The listing builds one solid part. Answer for the finished solid, in the listing's coordinates (mm). Face numbers are marked on the shaded views. A direction names the side the tool comes from. Give positions to 0.01 mm unless a question says otherwise; leave off trailing zeros. Loops run counter-clockwise (first coordinate to the right, second up) from the corner with the lowest first, then second, coordinate; pieces in that order, holes last. Notation, with made-up numbers: (-9.75, -36) - (38.25, -36) arc R30 cw to (38.25, -3) - close; hole circle Ø4 at (14, 28.25). An arc over 180 degrees is marked (long way). One line per item, written item: value. Start each with the question number.
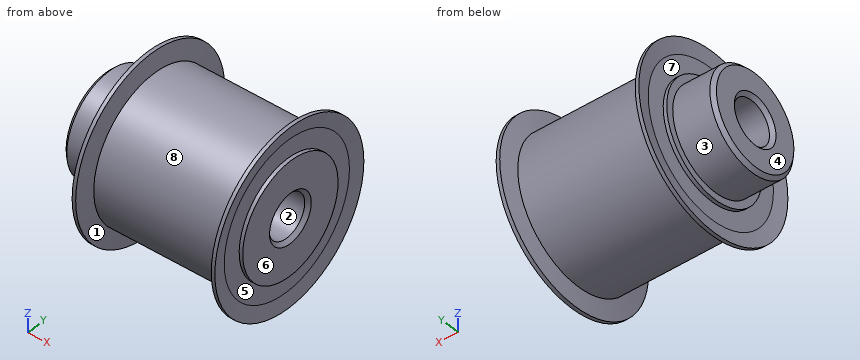
from build123d import *

# Parameters (mm, degrees)
FASE1_SIZE = 0.5


with BuildPart() as part:
    # Skizze1 → Rotation1 (revolve)
    with BuildSketch(Plane.XY, mode=Mode.PRIVATE) as rotation1_sk:
        Polygon((0, 3), (26, 3), (26, 8), (25.5, 8), (25.5, 10.5), (25.852653961, 12.5), (25.352653961, 12.5), (24.91183651, 10), (6.793471413, 10), (6.352653961, 12.5), (5.852653961, 12.5), (6.205307923, 10.5), (6.205307923, 8), (5.705307923, 8), (5.705307923, 7), (0, 7), align=None)
    revolve(rotation1_sk.sketch.rotate(Axis((0, 0, 0), (1, 0, 0)), 90), axis=Axis((0, 0, 0), (1, 0, 0)))

    # Fase1
    fase1_edges = [part.edges().sort_by_distance(p)[0] for p in [
        (0, 0, -3),
        (26, 0, -3),
        (0, 0, -7),
    ]]
    chamfer(fase1_edges, length=FASE1_SIZE)


solid = part.part
1. Find the intervals of material crossed by L1, parallel to Y at x = 5.75, z = 0; L2, parallel to Y at x = 19.5, z = 0; L3, parallel to X at y = 4, z = -9.5, in increasing order. Write a range as [from, to].
2. A cutting plane is placed at A-A (x = 15.75). Determine the outline of the cut face in (y, z), plus the area to 3 significant figures.
3. Determine the mould class of the marked faces 6, 7 and 8 for opening direction Z: released by +Z, released by -Z, zero draft, split by the parting line, or undercut.
4. Flat-ended cylindrical pins translate along their axes: pin 1 (1.5 mm diameter, centred on x = 10.5, y = -6, fed in from -Z); pin 2 (8 mm diameter, centred on x = 16.5, z = -1, fed in from -Y); pin 3 (3 mm diameter, centred on x = 8.5, y = 3.5, fed in from +Z); pin 4 (3.5 mm diameter, centred on y = 0, z = 0, fed in from -X). Find the tip coordinate at first contact, or state that the pin passes through.
5. A cutting plane is placed at B-B (x = 2.25). Determine the outline of the cut face in (y, z), plus the area to 3 significant figures.
6. For the marked faces 1, 2, 3, 4 and 5, determine the directions among +Z, -Z, +X, -X, +Y, -Y from which every point of the face is accessible in a straight line to the end or side of a thin tool.
Results below:
1. L1: y = [-8, -3], [3, 8]
1. L2: y = [-10, -3], [3, 10]
1. L3: x = [6.21, 6.74], [24.97, 25.5]
2. outline: circle Ø20 at (0, 0); hole circle Ø6 at (0, 0)
2. area: 286 mm^2
3. face 6: zero draft
3. face 7: undercut
3. face 8: split by the parting line
4. pin 1: stops at z = -8.51
4. pin 2: stops at y = -10
4. pin 3: stops at z = 9.8
4. pin 4: passes through
5. outline: circle Ø14 at (0, 0); hole circle Ø6 at (0, 0)
5. area: 126 mm^2
6. face 1: none
6. face 2: +X, -X
6. face 3: -X
6. face 4: +Z, -Z, -X, +Y, -Y
6. face 5: +X
